For this review, take the finished solid that the model builds, in its own axes (mm). A direction names the side the tool comes from. Give positions to 0.01 mm unless a question says otherwise; leave off trailing zeros. Loops run counter-clockwise (first coordinate to the right, second up) from the corner with the lowest first, then second, coordinate; pieces in that order, holes last.
Autodesk Inventor part; units mm, degrees
ref_plane "YZ Plane" through (0, 0, 0) normal (1, 0, 0) x (0, 1, 0)
ref_plane "XZ Plane" through (0, 0, 0) normal (0, 1, 0) x (-1, 0, 0)
ref_plane "XY Plane" through (0, 0, 0) normal (0, 0, 1) x (1, 0, 0)
sketch "Sketch1" plane through (0, 0, 0) normal (0, 0, 1) x (1, 0, 0)
  line L0 (0, 0) -> (25, 600)
  line L1 (25, 600) -> (375, 600)
  line L2 (375, 600) -> (400, 0)
  line L3 (400, 0) -> (0, 0)
  arc A0 (120.3096, 600) -> (279.6904, 600) centre (200, 673.1568) ccw
  line L4 (120.3096, 600) -> (25, 600)
  line L5 (25, 600) -> (0, 0)
  dimension "d0" = 600
  dimension "d1" = 25
  dimension "d2" = 350
  dimension "d3" = 400
  dimension "d4" = 175
extrude "Extrusion1" add sketch "Sketch1" along normal blind 50
fillet "Fillet1" radius 20 5 edges at (200, 600, 0) (387.5, 300, 0) (12.5, 300, 0) (25, 600, 25) (375, 600, 25)
fillet "Fillet2" radius 5 5 edges at (200, 600, 50) (30.3394, 594.4335, 50) (369.6606, 594.4335, 50) (387.8993, 290.4163, 50) (12.1007, 290.4163, 50)
sketch "Sketch2" plane through (0, 0, 0) normal (0, 0, 1) x (1, 0, 0)
  point P0 (0, 0)
sketch "Sketch3" plane through (0, 0, 0) normal (1, 0, 0) x (0, 1, 0)
  line L0 (0, 0) -> (0, 20)
  circle A0 centre (0, 20) radius 11.125
  dimension "d9" = 22.25
extrude "Extrusion2" add sketch "Sketch3" along normal blind 400
sketch "Sketch4" plane through (0, 0, 0) normal (0, 1, 0) x (-1, 0, 0)
  circle A0 centre (-325, 12.7) radius 11.5572
  circle A1 centre (-75, 12.7) radius 11.125
  line L0 (0, 31.125) -> (-400, 31.125)
  line L1 (-200, 31.125) -> (-350.8375, 31.125)
  point P0 (0, 0)
  dimension "d12" = 22.25
  dimension "d13" = 250
  dimension "d16" = 125
extrude "Extrusion3" add sketch "Sketch4" against normal blind 30
properties part number "backrest wheelchair EG26"
Q1. For pin 1 Ø8 at (x, z) = (168, 5.5) entering from +Y; pin 2 Ø15 at (x, z) = (181.5, 39) entering from -Y; pin 3 Ø1 at (x, z) = (157.5, 26.5) entering from -Y, all flat-tipped, find the tip position at first contact; note any pin that passes through.
Answers:
pin 1: stops at y = 597.02
pin 2: stops at y = 0
pin 3: stops at y = -9.37
Q2. Mouldability with a two-part tool opening along X and no side actions: class faces 1 (the cylindrical face through (30.495, 594.581, 32.675)), 2 (the cylindrical face through (319.667, -18.123, 2.447)), 3 (the flat face through (203, 0, 40)) as +X half, -X half, draft (parallel to the pull), parting line (faces both ways), or undercut.
Answers:
face 1: -X half
face 2: undercut
face 3: draft
Q3. Consider section A-A on x = 325. Give the boundary of the cut face in (y, z) (3 decimals).
Answers:
outline: (-30, 1.143) - (0, 1.143) - (0, 0) - (580, 0) arc R20 ccw to (600, 20) - (600, 45) arc R5 ccw to (595, 50) - (0, 50) - (0, 31.125) arc R11.125 ccw to (-10.278, 24.257) - (-30, 24.257) - close
Q4. Consider section B-B on x = 75. Give the boundary of the cut face in (y, z) (3 decimals), plus the area to 3 significant figures.
Answers:
outline: (-30, 1.575) - (0, 1.575) - (0, 0) - (580, 0) arc R20 ccw to (600, 20) - (600, 45) arc R5 ccw to (595, 50) - (0, 50) - (0, 31.125) arc R11.125 ccw to (-10.447, 23.825) - (-30, 23.825) - close
area: 30,600 mm2
Q5. For probe 1 along Y at (x, z) = (355.5, 19); probe 2 along X at (y, z) = (11, 27.5); probe 3 along Y at (x, z) = (136.5, 34.5), list the stretches that pass through material, from the lowest coordinate up.
Answers:
probe 1: y = -11.08 to 599.97
probe 2: x = 0.46 to 399.54
probe 3: y = 0 to 600
Q6. Machinability: for faces 4 (the cylindrical face through (77.41, -18.12, 1.84)), 5 (the flat face through (198, 600, 32)), which of the approach directions +Z, -Z, +X, -X, +Y, -Y give a long, thin tool a straight path to every point of the face, cutting with its end or side? Answer none if there is none.
Answers:
face 4: -Y
face 5: +Z, -Z, +X, -X, +Y
